Autodesk Fusion 360 part; units mm, degrees
sketch "Sketch1" plane through (0, 0, 0) normal (0, 0, 1) x (1, 0, 0)
  circle A0 centre (0, 0) radius 2.75
  line L0 (0.585, -2.05) -> (-0.585, -2.05)
  line L1 (-0.585, 0.885) -> (-0.585, 2.05)
  line L2 (-0.585, 2.05) -> (0.585, 2.05)
  line L3 (0.585, -0.885) -> (0.585, -2.05)
  line L4 (0.585, -2.05) -> (-0.585, 2.05) construction
  line L5 (-0.585, -2.05) -> (0.585, 2.05) construction
  line L6 (2.05, -0.585) -> (0.885, -0.585)
  line L7 (-2.05, -0.585) -> (-2.05, 0.585)
  line L8 (0.885, 0.585) -> (2.05, 0.585)
  line L9 (2.05, 0.585) -> (2.05, -0.585)
  line L10 (2.05, -0.585) -> (-2.05, 0.585) construction
  line L11 (-2.05, -0.585) -> (2.05, 0.585) construction
  arc A1 (0.885, -0.585) -> (0.585, -0.885) centre (0.885, -0.885) ccw
  line L12 (0.585, 2.05) -> (0.585, 0.885)
  arc A2 (0.585, 0.885) -> (0.885, 0.585) centre (0.885, 0.885) ccw
  line L13 (-2.05, 0.585) -> (-0.885, 0.585)
  line L14 (-2.05, -0.585) -> (-0.885, -0.585)
  arc A3 (-0.885, 0.585) -> (-0.585, 0.885) centre (-0.885, 0.885) ccw
  line L15 (-0.585, -0.885) -> (-0.585, -2.05)
  arc A4 (-0.585, -0.885) -> (-0.885, -0.585) centre (-0.885, -0.885) ccw
  point P0 (0.585, -0.585)
  dimension "d1" = 5.5
  dimension "d2" = 1.17
  dimension "d3" = 4.1
  dimension "d4" = 4.1
  dimension "d5" = 1.17
  dimension "d6" = 0.3
  dimension "d7" = 0.3
  dimension "d8" = 0.3
  dimension "d9" = 0.3
extrude "Extrude1" add sketch "Sketch1" along normal blind 3.3
sketch "Sketch2" plane through (0, 0, 0) normal (0, 0, -1) x (1, 0, 0)
  line L0 (-2.05, 0.585) -> (-0.885, 0.585)
  arc A0 (-0.885, 0.585) -> (-0.585, 0.885) centre (-0.885, 0.885) ccw
  line L1 (-0.585, 0.885) -> (-0.585, 2.05)
  line L2 (-0.585, 2.05) -> (0.585, 2.05)
  line L3 (0.585, 2.05) -> (0.585, 0.885)
  arc A1 (0.585, 0.885) -> (0.885, 0.585) centre (0.885, 0.885) ccw
  line L4 (0.885, 0.585) -> (2.05, 0.585)
  line L5 (2.05, 0.585) -> (2.05, -0.585)
  line L6 (2.05, -0.585) -> (0.885, -0.585)
  arc A2 (0.885, -0.585) -> (0.585, -0.885) centre (0.885, -0.885) ccw
  line L7 (0.585, -0.885) -> (0.585, -2.05)
  line L8 (0.585, -2.05) -> (-0.585, -2.05)
  line L9 (-0.585, -2.05) -> (-0.585, -0.885)
  arc A3 (-0.585, -0.885) -> (-0.885, -0.585) centre (-0.885, -0.885) ccw
  line L10 (-0.885, -0.585) -> (-2.05, -0.585)
  line L11 (-2.05, -0.585) -> (-2.05, 0.585)
  circle A4 centre (0, 0) radius 2.75
  line L12 (4, 4) -> (-4, 4)
  line L13 (-4, 4) -> (-4, -4)
  line L14 (-4, -4) -> (4, -4)
  line L15 (4, -4) -> (4, 4)
  line L16 (4, 4) -> (-4, -4) construction
  line L17 (-4, 4) -> (4, -4) construction
  dimension "d12" = 8
  dimension "d13" = 8
extrude "Extrude2" add sketch "Sketch2" along normal blind 1 contours L0 A0 L1 L2 L3 A1 L4 L5 L6 A2 L7 L8 L9 A3 L10 L11 | A4 | L12 L13 L14 L15
fillet "Fillet1" radius 0.25 1 edges at (-2.5639, -0.9944, 0)
fillet "Fillet2" radius 0.2 1 edges at (-2.5639, -0.9944, 3.3)
fillet "Fillet3" radius 0.2 16 edges at (1.4675, -0.585, 3.3) (0.6729, -0.6729, 3.3) (0.585, -1.4675, 3.3) (2.05, 0, 3.3) (0.585, 1.4675, 3.3) (0.6729, 0.6729, 3.3) (1.4675, 0.585, 3.3) (0, 2.05, 3.3) (-1.4675, 0.585, 3.3) (-0.6729, 0.6729, 3.3) (-0.585, 1.4675, 3.3) (-2.05, 0, 3.3) (-0.585, -1.4675, 3.3) (-0.6729, -0.6729, 3.3) (-1.4675, -0.585, 3.3) (0, -2.05, 3.3)
Model file for the job. Use its own axes, mm. A direction names the side the tool comes from. Coordinates: 2 decimals unless noted, no trailing zeros. Loops run counter-clockwise (first coordinate to the right, second up) from the corner with the lowest first, then second, coordinate; pieces in that order, holes last. Notation, with made-up numbers: (-30.5, 65.5) - (-17.5, 65.5) arc R37 ccw to (-17.5, 102.5) - close; hole circle Ø10 at (-8, 46.25). An arc over 180 degrees is marked (long way). Write item = value, one per line. Start each with the question number.
Item 1: Drop flat-ended pins along their axis: pin 1 Ø0.9 at (y, z) = (0, 1.5) entering from +X; pin 2 Ø0.6 at (x, z) = (-1.5, 2) entering from +Y; pin 3 Ø0.6 at (y, z) = (0, 1.5) entering from -X. Give the stop position or say it passes through.
Item 2: Wall check: probe 1 along Z at (x, y) = (-2.5, -3); probe 2 along X at (y, z) = (1.5, 1.2) (3 decimals); probe 3 along X at (y, z) = (2, 0.35) (3 decimals). Give the ranges that are in metal, low to high. Write a range as [from, to].
Item 3: 3-axis set-ups, long thin cutter, end or side, ignore diameter. For faces 4 (the face through (0, -2.05, 2)), 5 (the face through (-0.1, 4, -0.5)): which of +Z, -Z, +X, -X, +Y, -Y reach the whole face in a straight line?
Item 4: Saw through at B-B, the plane z = 2.35. List the corners of the cut face in (x, y) (3 decimals).
Item 5: Pull direction Y, two halves, no side cores. Call faces 1 (the face through (4, 0.1, -0.5)), 2 (the face through (-0.585, 1.5, 1.5)), 3 (the face through (0.1, -4, -0.5)): +Y half, -Y half, draft (parallel to the pull), parting line (faces both ways), or undercut.
Item 6: Saw through at D-D, the plane x = 3.25. List the corners of the cut face in (y, z), then the cut area to 3 significant figures.
Item 7: Saw through at A-A, the plane y = 0. List the corners of the cut face in (x, z), then the cut area to 3 significant figures.
Answers:
q1.pin_1 = 2.75
q1.pin_2 = 2.47
q1.pin_3 = -2.75
q2.probe_1 = [-1, 0]
q2.probe_2 = [-2.305, -0.585], [0.585, 2.305]
q2.probe_3 = [-1.887, -0.585], [0.585, 1.887]
q3.face_4 = +Z
q3.face_5 = +Z, -Z, +X, -X, +Y
q4.outline = circle Ø5.5 at (0, 0); hole (-2.05, -0.585) - (-0.885, -0.585) arc R0.3 cw to (-0.585, -0.885) - (-0.585, -2.05) - (0.585, -2.05) - (0.585, -0.885) arc R0.3 cw to (0.885, -0.585) - (2.05, -0.585) - (2.05, 0.585) - (0.885, 0.585) arc R0.3 cw to (0.585, 0.885) - (0.585, 2.05) - (-0.585, 2.05) - (-0.585, 0.885) arc R0.3 cw to (-0.885, 0.585) - (-2.05, 0.585) - close
q5.face_1 = draft
q5.face_2 = undercut
q5.face_3 = -Y half
q6.outline = (-4, -1) - (4, -1) - (4, 0) - (-4, 0) - close
q6.area = 8.00 mm2
q7.outline = (-4, -1) - (4, -1) - (4, 0) - (3, 0) arc R0.25 cw to (2.75, 0.25) - (2.75, 3.1) arc R0.2 ccw to (2.55, 3.3) - (2.25, 3.3) arc R0.2 ccw to (2.05, 3.1) - (2.05, 0) - (-2.05, 0) - (-2.05, 3.1) arc R0.2 ccw to (-2.25, 3.3) - (-2.55, 3.3) arc R0.2 ccw to (-2.75, 3.1) - (-2.75, 0.25) arc R0.25 cw to (-3, 0) - (-4, 0) - close
q7.area = 12.6 mm2
